Here's how the part is built. I have some questions about the finished solid (model axes, mm). Face numbers are marked on the shaded views. Coordinates: 2 decimals unless noted, no trailing zeros. Order: outer loops, then holes, each group sorted by start corner. A loop starts at its lowest first (then second) coordinate and runs counter-clockwise, first axis right, second up. Notation, with made-up numbers: M 34.25,-20 L 63.25,-20 A24 cw 63.25,0 Z; hole C 74,50 d4. An arc over 180 degrees is marked long. Answer as CSV lines item,"result". Start each with the question number.
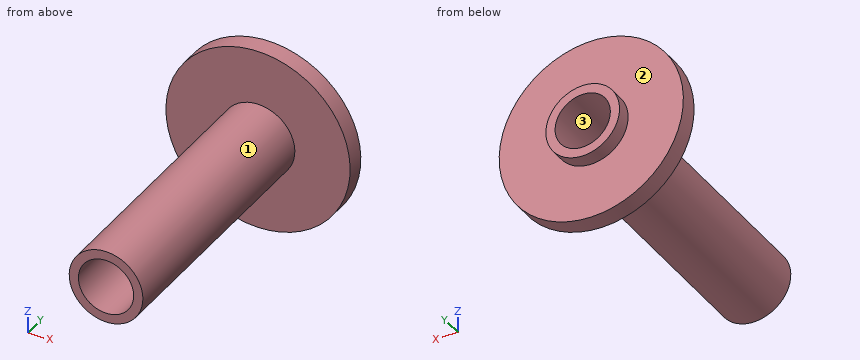
```python
from build123d import *

# Parameters (mm, degrees)
SKETCH1_R           = 10
SKETCH1_R_2         = 7.5
BOSS_EXTRUDE1_DEPTH = 80
SKETCH2_W           = 15
SKETCH2_H           = 5


with BuildPart() as part:
    # Sketch1 → Boss-Extrude1 (new body)
    with BuildSketch(Plane(origin=(0, 0, 0), x_dir=(1, 0, 0), z_dir=(0, 1, 0))):
        with Locations(Location((0, 0, 0), (0, 0, 270))):
            Circle(SKETCH1_R)
        with Locations(Location((0, 0, 0), (0, 0, 270))):
            Circle(SKETCH1_R_2, mode=Mode.SUBTRACT)
    extrude(amount=BOSS_EXTRUDE1_DEPTH)

    # Sketch2 → Revolve1 (revolve)
    with BuildSketch(Plane(origin=(0, 0, 0), x_dir=(0, 0, -1), z_dir=(1, 0, 0))):
        with Locations((17.5, 73.5)):
            Rectangle(SKETCH2_W, SKETCH2_H)
    revolve(axis=Axis((0, 0, 0), (0, 1, 0)))


solid = part.part
```
1) Suppose I cut it at B-B on x = 0. Please give me the cut outline in (y, z).
2) Suppose I cut it at A-A on z = 0. Please give me the cut outline in (x, y).
3) Suppose I cut it at D-D on x = -9. Please give me the cut outline in (y, z).
4) If we mould it in two halves opening along X, with no side actions, what happens to the marked faces 1, 2 and 3? For each: released by +X, released by -X, zero draft, split by the parting line, or undercut.
5) Suppose I cut it at C-C on y = 72.5. Please give me the cut outline in (x, z).
6) I need wall thicknesses on line 1 (X direction, y = 33.5, z = 0); line 2 (X direction, y = 71.5, z = -0.5) (3 decimals); line 3 (Y direction, x = 10, z = -2.5). Which ranges of each line are inside material? Lowest first, please. Write a range as [from, to].
7) Will these pins go through, and if not, where does the flat tip stop? pin 1 Ø15 at (x, z) = (8.5, -4) entering from -Y; pin 2 Ø12 at (y, z) = (40, -6.5) entering from +X; pin 3 Ø4 at (x, z) = (-4.5, -16) entering from -Y; pin 4 Ø12 at (x, y) = (5, 48) entering from +Z.
Output:
1,outline,"M 0,-10 L 71,-10 L 71,-25 L 76,-25 L 76,-10 L 80,-10 L 80,-7.5 L 0,-7.5 Z; M 0,7.5 L 80,7.5 L 80,10 L 76,10 L 76,25 L 71,25 L 71,10 L 0,10 Z"
2,outline,"M -25,71 L -10,71 L -10,0 L -7.5,0 L -7.5,80 L -10,80 L -10,76 L -25,76 Z; M 7.5,0 L 10,0 L 10,71 L 25,71 L 25,76 L 10,76 L 10,80 L 7.5,80 Z"
3,outline,"M 0,-4.36 L 71,-4.36 L 71,-23.32 L 76,-23.32 L 76,-4.36 L 80,-4.36 L 80,4.36 L 76,4.36 L 76,23.32 L 71,23.32 L 71,4.36 L 0,4.36 Z"
4,face 1,"split by the parting line"
4,face 2,"zero draft"
4,face 3,"undercut"
5,outline,"C 0,0 d50; hole C 0,0 d15"
6,line 1,"[-10, -7.5], [7.5, 10]"
6,line 2,"[-24.995, -7.483], [7.483, 24.995]"
6,line 3,"[71, 76]"
7,pin 1,"y = 0"
7,pin 2,"x = 9.99"
7,pin 3,"y = 71"
7,pin 4,"z = 10"
